Part model, mm, in its own coordinate system. A direction names the side the tool comes from. Give positions to 0.01 mm unless a question says otherwise; leave off trailing zeros. Write each loop counter-clockwise with the first axis right and the second up, starting at its lowest first coordinate (ties: lowest second). Pieces come first, ordered by that corner, then holes. Notation, with made-up numbers: M 34.25,-9 L 46.25,-9 A12 cw 46.25,11 Z; hole C 63.5,24.5 d9. An arc over 180 degrees is marked long. Use CSV: the item, a comma, the result in double quotes. Start each with the question number.
Item 1: Which spindle directions (+Z, -Z, +X, -X, +Y, -Y) get a long thin tool onto all of the face, cutting with end or side? Do faces 1 (the flat face through (-20, 2, 45)), 2 (the flat face through (-31, 5, 37)), 3 (the flat face through (71, 5, 37)). Say none if no direction does.
Item 2: Cut at D-D (y = 1.23). Count the separate pieces of the cut face and the enclosed holes in it, then the cut area to 3 significant figures.
Item 3: Cut at B-B (x = 7.5). List the corners of the cut face in (y, z).
Item 4: Pin check, flat tips, straight feed: pin 1 (3 mm diameter, centred on x = 32.5, z = 15, fed in from -Y); pin 2 (3.5 mm diameter, centred on y = -2.475, z = 59, fed in from +X); pin 3 (0.9 mm diameter, centred on x = -1.5, y = 1, fed in from -Z); pin 4 (2.5 mm diameter, centred on x = -30.5, y = 7, fed in from -Z). Stop position of each tip, or through.
Item 5: Cut at C-C (y = 7.5). List the corners of the cut face in (x, z).
Item 6: Mould opens along X. For faces 4 (the flat face through (-31.5, -11, 40)), 5 (the cylindrical face through (-1.521, 0.824, 43.812)), 6 (the flat face through (20, 6, 63)) say: released by +X, released by -X, zero draft, split by the parting line, or undercut.
Item 7: Cut at A-A (z = 15). List the corners of the cut face in (x, y), then the cut area to 3 significant figures.
Item 8: Drill centre lines: line 1 (X direction, y = 1, z = 48.5); line 2 (Y direction, x = -32, z = 59) (3 decimals); line 3 (X direction, y = -1, z = 44). Where is each one in solid material? Low to high. Write a range as [from, to].
from build123d import *

# Parameters (mm, degrees)
SKETCH1_W           = 40
SKETCH1_H           = 27
SKETCH1_R           = 1.9
BOSS_EXTRUDE3_DEPTH = 10
SKETCH5_W           = 100
SKETCH5_H           = 36
BOSS_EXTRUDE4_DEPTH = 10
SKETCH6_W           = 36
SKETCH6_H           = 32.65
SKETCH6_R           = 1.35
SKETCH6_R_2         = 6
BOSS_EXTRUDE6_DEPTH = 3
SKETCH7_W           = 80
SKETCH7_H           = 10
CUT_EXTRUDE1_DEPTH  = 36
SKETCH8_W           = 3
SKETCH8_H           = 6.3
BOSS_EXTRUDE7_DEPTH = 21
SKETCH10_R          = 1.35
CUT_EXTRUDE3_DEPTH  = 46
SKETCH11_R          = 3.75
CUT_EXTRUDE4_DEPTH  = 1.5
SKETCH12_W          = 10
SKETCH12_H          = 10
CUT_EXTRUDE5_DEPTH  = 5


with BuildPart() as part:
    # Sketch1 → Boss-Extrude3 (new body)
    with BuildSketch(Plane(origin=(0, 0, 0), x_dir=(1, 0, 0), z_dir=(0, 1, 0))):
        with Locations((20, -13.5)):
            Rectangle(SKETCH1_W, SKETCH1_H)
        with Locations(Location((7.5, -5, 0), (0, 0, 270))):
            Circle(SKETCH1_R, mode=Mode.SUBTRACT)
        with Locations(Location((7.5, -15, 0), (0, 0, 270))):
            Circle(SKETCH1_R, mode=Mode.SUBTRACT)
        with Locations(Location((32.5, -15, 0), (0, 0, 90))):
            Circle(SKETCH1_R, mode=Mode.SUBTRACT)
        with Locations(Location((32.5, -5, 0), (0, 0, 90))):
            Circle(SKETCH1_R, mode=Mode.SUBTRACT)
    extrude(amount=BOSS_EXTRUDE3_DEPTH)

    # Sketch5 → Boss-Extrude4 (add)
    with BuildSketch(Plane(origin=(0, 10, 0), x_dir=(1, 0, 0), z_dir=(0, 1, 0))):
        with Locations((20, -45)):
            Rectangle(SKETCH5_W, SKETCH5_H)
    extrude(amount=-BOSS_EXTRUDE4_DEPTH)

    # Sketch6 → Boss-Extrude6 (add)
    with BuildSketch(Plane(origin=(70, 0, 0), x_dir=(0, 0, -1), z_dir=(1, 0, 0))):
        with Locations((-45, -6.325)):
            Rectangle(SKETCH6_W, SKETCH6_H)
        with Locations((-59, -20.175)):
            Circle(SKETCH6_R, mode=Mode.SUBTRACT)
        with Locations((-59, -2.475)):
            Circle(SKETCH6_R, mode=Mode.SUBTRACT)
        with Locations(Location((-31, -20.175, 0), (0, 0, 180))):
            Circle(SKETCH6_R, mode=Mode.SUBTRACT)
        with Locations(Location((-31, -2.475, 0), (0, 0, 180))):
            Circle(SKETCH6_R, mode=Mode.SUBTRACT)
        with Locations((-51.4, -11.325)):
            Circle(SKETCH6_R_2, mode=Mode.SUBTRACT)
    boss_extrude6 = extrude(amount=BOSS_EXTRUDE6_DEPTH)

    # Mirror1: Boss-Extrude6 across plane
    add(boss_extrude6.mirror(Plane(origin=(20, 0, 0), x_dir=(0, 0, 1), z_dir=(1, 0, 0))))

    # Sketch7 → Cut-Extrude1 (cut)
    with BuildSketch(Plane.XY.offset(63)):
        with Locations((20, 0)):
            Rectangle(SKETCH7_W, SKETCH7_H)
    extrude(amount=-CUT_EXTRUDE1_DEPTH, mode=Mode.SUBTRACT)

    # Sketch8 → Boss-Extrude7 (add)
    with BuildSketch(Plane.XY.offset(63)):
        with Locations((-1.5, 1.85)):
            Rectangle(SKETCH8_W, SKETCH8_H)
    boss_extrude7 = extrude(amount=-BOSS_EXTRUDE7_DEPTH)

    # Mirror2: Boss-Extrude7 across plane
    add(boss_extrude7.mirror(Plane(origin=(20, 0, 0), x_dir=(0, 0, 1), z_dir=(1, 0, 0))))

    # Sketch10 → Cut-Extrude3 (cut)
    with BuildSketch(Plane.ZY.offset(3)):
        with Locations(Location((57.7, 1.23, 0), (0, 0, 270))):
            Circle(SKETCH10_R)
        with Locations(Location((45.1, 1.23, 0), (0, 0, 180))):
            Circle(SKETCH10_R)
    extrude(amount=-CUT_EXTRUDE3_DEPTH, mode=Mode.SUBTRACT)

    # Sketch11 → Cut-Extrude4 (cut)
    with BuildSketch(Plane(origin=(-30, 0, 0), x_dir=(0, 0, -1), z_dir=(1, 0, 0))):
        with Locations((-39.95, -11.325)):
            Circle(SKETCH11_R)
    cut_extrude4 = extrude(amount=-CUT_EXTRUDE4_DEPTH, mode=Mode.SUBTRACT)

    # Mirror3: Cut-Extrude4 across plane
    add(cut_extrude4.mirror(Plane(origin=(20, 0, 0), x_dir=(0, 0, 1), z_dir=(1, 0, 0))), mode=Mode.SUBTRACT)

    # Sketch12 → Cut-Extrude5 (cut)
    with BuildSketch(Plane(origin=(73, 0, 0), x_dir=(0, 0, -1), z_dir=(1, 0, 0))):
        with Locations((-32, 5)):
            Rectangle(SKETCH12_W, SKETCH12_H)
    cut_extrude5 = extrude(amount=-CUT_EXTRUDE5_DEPTH, mode=Mode.SUBTRACT)

    # Mirror4: Cut-Extrude5 across plane
    add(cut_extrude5.mirror(Plane(origin=(20, 0, 0), x_dir=(0, 0, 1), z_dir=(1, 0, 0))), mode=Mode.SUBTRACT)


solid = part.part
Worked answers:
1,face 1,"+Z, -Z, -Y"
1,face 2,"-Z, -X, +Y"
1,face 3,"-Z, +X, +Y"
2,separate pieces,"9"
2,enclosed holes,"4"
2,area,"1,960 mm^2"
3,outline,"M 0,0 L 10,0 L 10,3.1 L 0,3.1 Z; M 0,6.9 L 10,6.9 L 10,13.1 L 0,13.1 Z; M 0,16.9 L 10,16.9 L 10,63 L 5,63 L 5,27 L 0,27 Z"
4,pin 1,"passes through"
4,pin 2,"stops at x = 73"
4,pin 3,"stops at z = 42"
4,pin 4,"stops at z = 37"
5,outline,"M -33,37 L -28,37 L -28,27 L 0,27 L 0,0 L 40,0 L 40,27 L 68,27 L 68,37 L 73,37 L 73,63 L -33,63 Z; hole C 7.5,5 d3.8; hole C 7.5,15 d3.8; hole C 32.5,5 d3.8; hole C 32.5,15 d3.8"
6,face 4,"undercut"
6,face 5,"undercut"
6,face 6,"zero draft"
7,outline,"M 0,0 L 5.6,0 L 5.6,10 L 0,10 Z; M 9.4,0 L 30.6,0 L 30.6,10 L 9.4,10 Z; M 34.4,0 L 40,0 L 40,10 L 34.4,10 Z"
7,area,"324 mm^2"
8,line 1,"x = [-33, -20], [-3, 0], [40, 43], [60, 73]"
8,line 2,"y = [-22.65, -21.525], [-18.825, -3.825], [-1.125, 10]"
8,line 3,"x = [-33, -30], [-3, 0], [40, 43], [70, 73]"
